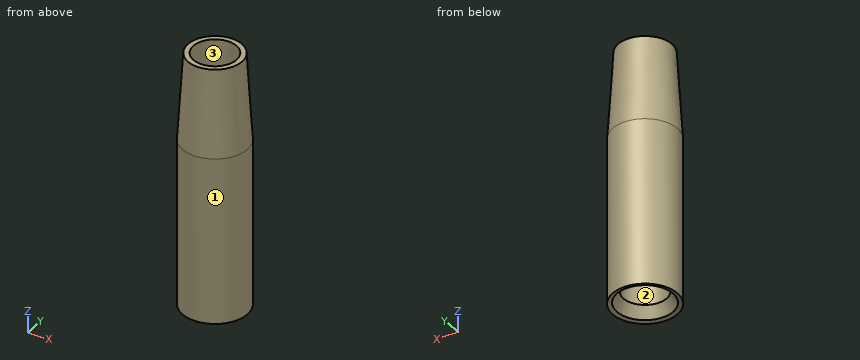
from build123d import *

# Parameters (mm, degrees)
SKETCH_1_R          = 15
EXTRUDE_1_DEPTH     = 77
SKETCH_3_R          = 12.5
SKETCH_2_R          = 15
SKETCH_5_R          = 10
CUT_EXTRUDE_1_DEPTH = 60
CUT_EXTRUDE_START   = -40.5
SKETCH_6_R          = 10
CUT_EXTRUDE_2_DEPTH = 40.5
CHAMFER_1_SIZE      = 3.5
CHAMFER_1_SIZE2     = 6.062177826
CHAMFER_2_SIZE      = 2.732050808
CHAMFER_2_SIZE_2    = 1


with BuildPart() as part:
    # 스케치1 → 보스-돌출1 (new body)
    with BuildSketch(Plane.XY):
        Circle(SKETCH_1_R)
    extrude(amount=EXTRUDE_1_DEPTH)

    # 스케치3 → 로프트1 section 0
    with BuildSketch(Plane.XY.offset(117)):
        Circle(SKETCH_3_R)
    # 스케치2 → 로프트1 section 1
    with BuildSketch(Plane.XY.offset(77)):
        Circle(SKETCH_2_R)
    loft()

    # 스케치5 → 컷-돌출1 (cut)
    with BuildSketch(Plane.XY.offset(117)):
        Circle(SKETCH_5_R)
    extrude(amount=-CUT_EXTRUDE_1_DEPTH, mode=Mode.SUBTRACT)

    # 스케치6 → 컷-돌출2 (cut)
    with BuildSketch(Plane(origin=(0, 0, 0), x_dir=(-1, 0, 0), z_dir=(0, 0, -1)).offset(CUT_EXTRUDE_START)):
        with Locations(Location((0, 0, 0), (0, 0, 180))):
            Circle(SKETCH_6_R)
    extrude(amount=CUT_EXTRUDE_2_DEPTH, mode=Mode.SUBTRACT)

    # 모따기1
    chamfer_1_edges = [part.edges().sort_by_distance(p)[0] for p in [
        (-10, 0, 0),
    ]]
    chamfer_1_side = [part.faces().sort_by_distance(p)[0] for p in [
        (-14.575735931, 0, 0),
    ]]
    chamfer(chamfer_1_edges, length=CHAMFER_1_SIZE, length2=CHAMFER_1_SIZE2, reference=chamfer_1_side[0])

    # 모따기2
    # the kernel refuses this chamfer: 2.732050808, 1 mm, written as the material it takes off along each edge
    with BuildSketch(Plane(origin=(0, 0, 0), x_dir=(1, 0, 0), z_dir=(0, 1, 0))) as chamfer_2_piece_1:
        Polygon((13.5 + CHAMFER_2_SIZE, 0), (13.5 - CHAMFER_2_SIZE_2 * 0.5, -CHAMFER_2_SIZE_2 * 0.866025403784), (13.5, 0), align=None)
    revolve(axis=Axis((0, 0, 0), (0, 0, -1)), mode=Mode.SUBTRACT)


solid = part.part
Geometry: final body of the model. Coordinates: model frame, mm. Face numbers are marked on the shaded views. A direction names the side the tool comes from. Round coordinates to 2 decimals unless told otherwise and drop trailing zeros. Order: outer loops, then holes, each group sorted by start corner. A loop starts at its lowest first (then second) coordinate and runs counter-clockwise, first axis right, second up.
Q1. Material intervals for probe 1 along Y at (x, z) = (0, 24); probe 2 along Z at (x, y) = (1.5, -4); probe 3 along X at (y, z) = (-7, 26.5), sorted ascending.
Result sheet:
probe 1: y = -15 to -10, 10 to 15
probe 2: z = 40.5 to 57
probe 3: x = -13.27 to -7.14, 7.14 to 13.27
Q2. Section A-A, the plane x = 0. Output: boundary loops of the cut face in (y, z).
Result sheet:
outline: (-15, 0.33) - (-13, 0.87) - (-10, 6.06) - (-10, 40.5) - (10, 40.5) - (10, 6.06) - (13, 0.87) - (15, 0.33) - (15, 77) - (12.5, 117) - (10, 117) - (10, 57) - (-10, 57) - (-10, 117) - (-12.5, 117) - (-15, 77) - close
Q3. Section B-B, the plane z = 48. Output: boundary loops of the cut face in (x, y).
Result sheet:
outline: circle Ø30 at (0, 0)
Q4. Section D-D, the plane z = 93.5. Output: boundary loops of the cut face in (x, y).
Result sheet:
outline: circle Ø27.94 at (0, 0); hole circle Ø20 at (0, 0)
Q5. Access query for the marked faces 1, 2 and 3. Directions: +Z, -Z, +X, -X, +Y, -Y. A direction counts if a zero-diameter tool reaches every point of the face in a straight line with its end or side. Return the directions, or none.
Result sheet:
face 1: +Z, -Z
face 2: -Z
face 3: +Z
Q6. Section C-C, the plane z = 68. Output: boundary loops of the cut face in (x, y).
Result sheet:
outline: circle Ø30 at (0, 0); hole circle Ø20 at (0, 0)
Q7. Pin query (flat end, axial travel): pin 1 (6 mm diameter, centred on x = 4.5, y = -1, fed in from -Z); pin 2 (12 mm diameter, centred on x = -8.5, z = 33, fed in from +Y); pin 3 (6 mm diameter, centred on x = 10, z = 101, fed in from -Y). Return the tip coordinate at first contact, or that it passes through.
Result sheet:
pin 1: stops at z = 40.5
pin 2: stops at y = 14.79
pin 3: stops at y = -11.56
